Work out the finished part from the listing and answer in its coordinate system (mm). Coordinates: 2 decimals unless noted, no trailing zeros. Loops run counter-clockwise (first coordinate to the right, second up) from the corner with the lowest first, then second, coordinate; pieces in that order, holes last.
```python
from build123d import *

# Parameters (mm, degrees)
SKETCH1_W           = 232.41
SKETCH1_H           = 38.1
SKETCH1_R           = 6.35
BOSS_EXTRUDE1_DEPTH = 4.7625


with BuildPart() as part:
    # Sketch1 → Boss-Extrude1 (new body)
    with BuildSketch(Plane.XY):
        with Locations((116.205, 19.05)):
            Rectangle(SKETCH1_W, SKETCH1_H)
        with Locations(Location((38.4175, 19.05, 0), (0, 0, 180))):
            Circle(SKETCH1_R, mode=Mode.SUBTRACT)
        with Locations(Location((193.9925, 19.05, 0), (0, 0, 180))):
            Circle(SKETCH1_R, mode=Mode.SUBTRACT)
        with Locations(Location((139.7, 19.05, 0), (0, 0, 180))):
            Circle(SKETCH1_R, mode=Mode.SUBTRACT)
    extrude(amount=BOSS_EXTRUDE1_DEPTH)


solid = part.part
```
1. Straight lines are drawn through the part: probe 1 along X at (y, z) = (19.05, 1.85); probe 2 along Y at (x, z) = (139.7, 3.75); probe 3 along X at (y, z) = (23.5, 3.75). For each, find the intervals that lie inside material, in ascending order.
2. A cutting plane is placed at A-A, the plane y = 19.05. Give the vertices of the cut face in (x, z), then the cut area to 3 significant figures.
3. A cutting plane is placed at C-C, the plane z = 2.9. Give the vertices of the cut face in (x, y), then the cut area to 3 significant figures.
4. A cutting plane is placed at B-B, the plane x = 139.7. Give the vertices of the cut face in (y, z).
5. Determine the mould class of faces 1 (the cylindrical face through (146.044, 18.771, 2.348)), 2 (the flat face through (115, 19, 0)), 3 (the flat face through (232.41, 19, 2)) for opening direction X: released by +X, released by -X, zero draft, split by the parting line, or undercut.
Answers below:
1. probe 1: x = 0 to 32.07, 44.77 to 133.35, 146.05 to 187.64, 200.34 to 232.41
1. probe 2: y = 0 to 12.7, 25.4 to 38.1
1. probe 3: x = 0 to 33.89, 42.95 to 135.17, 144.23 to 189.46, 198.52 to 232.41
2. outline: (0, 0) - (32.07, 0) - (32.07, 4.76) - (0, 4.76) - close; (44.77, 0) - (133.35, 0) - (133.35, 4.76) - (44.77, 4.76) - close; (146.05, 0) - (187.64, 0) - (187.64, 4.76) - (146.05, 4.76) - close; (200.34, 0) - (232.41, 0) - (232.41, 4.76) - (200.34, 4.76) - close
2. area: 925 mm2
3. outline: (0, 0) - (232.41, 0) - (232.41, 38.1) - (0, 38.1) - close; hole circle Ø12.7 at (38.42, 19.05); hole circle Ø12.7 at (139.7, 19.05); hole circle Ø12.7 at (193.99, 19.05)
3. area: 8,470 mm2
4. outline: (0, 0) - (12.7, 0) - (12.7, 4.76) - (0, 4.76) - close; (25.4, 0) - (38.1, 0) - (38.1, 4.76) - (25.4, 4.76) - close
5. face 1: undercut
5. face 2: zero draft
5. face 3: released by +X
